Input: dimensioned drawing with shaded views. Units: mm. Origin: part minimum x, y, z. A direction names the side the tool comes from. Round coordinates to 2 decimals unless told otherwise and drop trailing zeros. Loops run counter-clockwise (first coordinate to the right, second up) from the corner with the lowest first, then second, coordinate; pieces in that order, holes last.
1) First-contact query: pin 1 (1 mm diameter, centred on x = 44.5, y = 24.5, fed in from +Z); pin 2 (9 mm diameter, centred on x = 78, y = 23, fed in from -Z); pin 3 (10 mm diameter, centred on x = 10.5, y = 36, fed in from -Z). Flat tips, straight axial feed; report the tip coordinate or a pass-through.
2) Section C-C, the plane y = 20. Return loops of the section in (x, z), and give its area (3 significant figures).
3) Section B-B, the plane x = 17.5. Return loops of the section in (y, z), and give its area (3 significant figures).
4) Access query for the marked faces 4, 5 and 6. Directions: +Z, -Z, +X, -X, +Y, -Y. A direction counts if a zero-diameter tool reaches every point of the face in a straight line with its end or side. Return the directions, or none.
5) Section D-D, the plane z = 55. Return loops of the section in (x, y).
6) Draft query along X for the marked faces 1, 2 and 3. Return one class per face: pulls with the +X half, pulls with the -X half, needs draft (parallel to the pull), parting line crosses it, or undercut.
7) Ray query, line 1 along X through (y, z) = (20, 8.75); line 2 along Y through (x, z) = (17, 9); line 3 along Z through (x, y) = (64, 7). Return the intervals inside material, ascending.
8) Section A-A, the plane z = 13.5. Return loops of the section in (x, y), and give its area (3 significant figures).
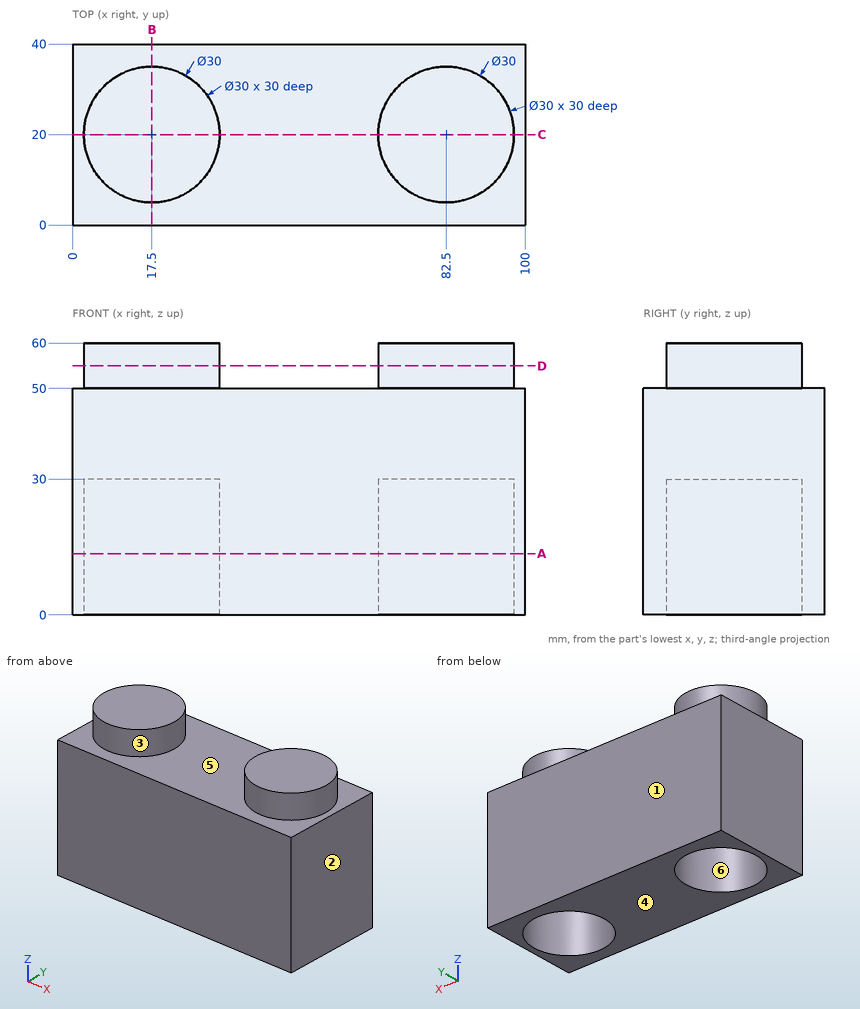
Final values:
1. pin 1: stops at z = 50
1. pin 2: stops at z = 30
1. pin 3: stops at z = 0
2. outline: (0, 0) - (2.5, 0) - (2.5, 30) - (32.5, 30) - (32.5, 0) - (67.5, 0) - (67.5, 30) - (97.5, 30) - (97.5, 0) - (100, 0) - (100, 50) - (97.5, 50) - (97.5, 60) - (67.5, 60) - (67.5, 50) - (32.5, 50) - (32.5, 60) - (2.5, 60) - (2.5, 50) - (0, 50) - close
2. area: 3,800 mm2
3. outline: (0, 0) - (5, 0) - (5, 30) - (35, 30) - (35, 0) - (40, 0) - (40, 50) - (35, 50) - (35, 60) - (5, 60) - (5, 50) - (0, 50) - close
3. area: 1,400 mm2
4. face 4: -Z, +X, -X, +Y, -Y
4. face 5: +Z
4. face 6: -Z
5. outline: circle Ø30 at (17.5, 20); circle Ø30 at (82.5, 20)
6. face 1: needs draft
6. face 2: pulls with the +X half
6. face 3: undercut
7. line 1: x = 0 to 2.5, 32.5 to 67.5, 97.5 to 100
7. line 2: y = 0 to 5.01, 34.99 to 40
7. line 3: z = 0 to 50
8. outline: (0, 0) - (100, 0) - (100, 40) - (0, 40) - close; hole circle Ø30 at (17.5, 20); hole circle Ø30 at (82.5, 20)
8. area: 2,590 mm2
